Source: CAD feature listing. Evaluate the final solid. Frame: model axes, mm. Face numbers are marked on the shaded views. A direction names the side the tool comes from. Give positions to 0.01 mm unless a question says otherwise; leave off trailing zeros. Order: outer loops, then holes, each group sorted by start corner. A loop starts at its lowest first (then second) coordinate and runs counter-clockwise, first axis right, second up.
from build123d import *

# Parameters (mm, degrees)
SKETCH1_R           = 1.1
BOSS_EXTRUDE1_DEPTH = 20
SKETCH2_W           = 8.5
SKETCH2_H           = 70
SKETCH2_W_2         = 17.75
SKETCH2_H_2         = 26
BOSS_EXTRUDE2_DEPTH = 1.25
CUT_EXTRUDE1_START  = -10
CUT_EXTRUDE1_DEPTH  = 1.8


with BuildPart() as part:
    # Sketch1 → Boss-Extrude1 (new body)
    with BuildSketch(Plane(origin=(0, 0, 0), x_dir=(1, 0, 0), z_dir=(0, 1, 0))):
        with BuildLine():
            Line((-30, 0), (-30, -60))
            Line((-30, -60), (30, -60))
            Line((30, -60), (30, 0))
            ThreePointArc((30, 0), (0, 30), (-30, 0))
        make_face()
        with Locations((27.94, 0)):
            Circle(SKETCH1_R, mode=Mode.SUBTRACT)
        with Locations((-27.94, 0)):
            Circle(SKETCH1_R, mode=Mode.SUBTRACT)
        with Locations((0, 27.94)):
            Circle(SKETCH1_R, mode=Mode.SUBTRACT)
        with Locations((-27.94, -57.785)):
            Circle(SKETCH1_R, mode=Mode.SUBTRACT)
        with Locations((27.94, -57.785)):
            Circle(SKETCH1_R, mode=Mode.SUBTRACT)
        with BuildLine():
            Line((27.94, -55.785), (27.94, -2))
            ThreePointArc((27.94, -2), (25.940320377, -0.035796715), (27.868418039, 1.998718595))
            ThreePointArc((27.868418039, 1.998718595), (19.756563466, 19.756563466), (1.998718595, 27.868418039))
            ThreePointArc((1.998718595, 27.868418039), (0, 25.94), (-1.998718595, 27.868418039))
            ThreePointArc((-1.998718595, 27.868418039), (-19.756563466, 19.756563466), (-27.868418039, 1.998718595))
            ThreePointArc((-27.868418039, 1.998718595), (-25.940320377, -0.035796715), (-27.94, -2))
            Line((-27.94, -2), (-27.94, -55.785))
            ThreePointArc((-27.94, -55.785), (-26.525786438, -56.370786438), (-25.94, -57.785))
            Line((-25.94, -57.785), (25.94, -57.785))
            ThreePointArc((25.94, -57.785), (26.525786438, -56.370786438), (27.94, -55.785))
        make_face(mode=Mode.SUBTRACT)
    extrude(amount=-BOSS_EXTRUDE1_DEPTH)

    # Sketch2 → Boss-Extrude2 (add)
    with BuildSketch(Plane.XZ.offset(20)):
        with BuildLine():
            Line((30, 0), (30, 60))
            Line((30, 60), (-30, 60))
            Line((-30, 60), (-30, 0))
            ThreePointArc((-30, 0), (0, -30), (30, 0))
        make_face()
        Polygon((-7.25, 53), (-7.25, 32), (-25, 32), (-25, 55), (-7.25, 55), align=None, mode=Mode.SUBTRACT)
        with Locations((0, 15)):
            Rectangle(SKETCH2_W, SKETCH2_H, mode=Mode.SUBTRACT)
        Polygon((7.25, 53), (7.25, 32), (25, 32), (25, 55), (7.25, 55), align=None, mode=Mode.SUBTRACT)
        with Locations((16.125, 15)):
            Rectangle(SKETCH2_W_2, SKETCH2_H_2, mode=Mode.SUBTRACT)
        with BuildLine():
            Line((-7.25, -16.347418764), (-9.399268665, -23.165788322))
            ThreePointArc((-9.399268665, -23.165788322), (-20.160567843, -14.783487553), (-24.919871589, -2))
            Line((-24.919871589, -2), (-7.25, -2))
            Line((-7.25, -2), (-7.25, -16.347418764))
        make_face(mode=Mode.SUBTRACT)
        with BuildLine():
            Line((7.25, -16.347418764), (9.399268665, -23.165788322))
            ThreePointArc((9.399268665, -23.165788322), (20.160567843, -14.783487553), (24.919871589, -2))
            Line((24.919871589, -2), (7.25, -2))
            Line((7.25, -2), (7.25, -16.347418764))
        make_face(mode=Mode.SUBTRACT)
        with Locations((-16.125, 15)):
            Rectangle(SKETCH2_W_2, SKETCH2_H_2, mode=Mode.SUBTRACT)
    extrude(amount=-BOSS_EXTRUDE2_DEPTH)

    # Sketch3 → Cut-Extrude1 (cut)
    with BuildSketch(Plane(origin=(0, 0, 0), x_dir=(1, 0, 0), z_dir=(0, 1, 0)).offset(CUT_EXTRUDE1_START)):
        Polygon((2.424871131, 27.94), (1.212435565, 30.04), (-1.212435565, 30.04), (-2.424871131, 27.94), (-2.923440006, 27.076453377), (-1.212435565, 25.84), (1.212435565, 25.84), (2.664841123, 27.524359781), align=None)
        Polygon((27.94, -2.424871131), (30.04, -1.212435565), (30.04, 1.212435565), (27.94, 2.424871131), (27.29756517, 2.795781052), (25.84, 1.212435565), (25.84, -1.212435565), align=None)
        Polygon((30.28224565, -58.412602831), (29.65464282, -56.07035718), (27.312397169, -55.44275435), (25.59775435, -57.157397169), (26.22535718, -59.49964282), (28.567602831, -60.12724565), (30.909848481, -60.754848481), align=None)
        Polygon((-25.59775435, -57.157397169), (-27.312397169, -55.44275435), (-29.65464282, -56.07035718), (-30.28224565, -58.412602831), (-30.909848481, -60.754848481), (-28.567602831, -60.12724565), (-26.22535718, -59.49964282), align=None)
        Polygon((-30.04, 1.212435565), (-30.04, -1.212435565), (-27.94, -2.424871131), (-25.84, -1.212435565), (-25.84, 1.212435565), (-27.443113573, 2.711748643), (-27.94, 2.424871131), align=None)
    extrude(amount=-CUT_EXTRUDE1_DEPTH, mode=Mode.SUBTRACT)


solid = part.part
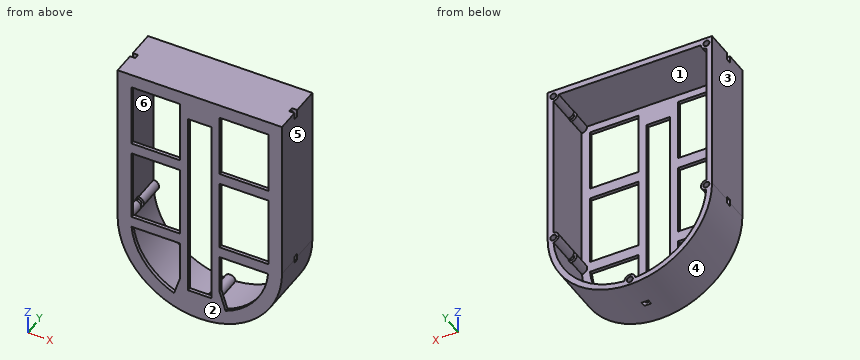
(1) Section C-C, the plane y = -5.25. Return loops of the section in (x, z) (3 decimals).
(2) Section B-B, the plane x = 0. Return loops of the section in (y, z) (3 decimals).
(3) Section D-D, the plane z = -18. Return loops of the section in (x, y), plus the area to 3 significant figures.
(4) Access query for the marked faces 5 and 6. Directions: +Z, -Z, +X, -X, +Y, -Y. A direction counts if a zero-diameter tool reaches every point of the face in a straight line with its end or side. Return the directions, or none.
(5) Line query: line 1 along X through (y, z) = (-3.25, 0); line 2 along Z through (x, y) = (0, -7.75) (3 decimals); line 3 along X through (y, z) = (-18.5, 10.5). Output: solid intervals per line, ascending.
(6) Pin query (flat end, axial travel): pin 1 Ø5.5 at (x, y) = (-2, -10.5) entering from -Z; pin 2 Ø3 at (x, z) = (-27.94, 57.785) entering from +Y; pin 3 Ø1.1 at (x, z) = (-28, 57.5) entering from +Y; pin 4 Ø2 at (x, y) = (-9.5, -6.5) entering from -Z. Return the tip coordinate at first contact, or that it passes through.
(7) Section A-A, the plane z = 13. Return loops of the section in (x, y).
(8) Draft query along X for the marked faces 1, 2, 3 and 4. Return one class per face: +X half, -X half, draft (parallel to the pull), parting line (faces both ways), or undercut.
Checks:
1. outline: (-30, 0) arc R30 ccw to (30, 0) - (30, 60) - (-30, 60) - close; hole circle Ø2.2 at (-27.94, 0); hole circle Ø2.2 at (-27.94, 57.785); hole (-27.94, 2) arc R2 cw to (-27.868, -1.999) arc R27.94 ccw to (-1.999, -27.868) arc R2 cw to (1.999, -27.868) arc R27.94 ccw to (27.868, -1.999) arc R2 cw to (27.94, 2) - (27.94, 55.785) arc R2 cw to (25.94, 57.785) - (-25.94, 57.785) arc R2 cw to (-27.94, 55.785) - close; hole circle Ø2.2 at (0, -27.94); hole circle Ø2.2 at (27.94, 0); hole circle Ø2.2 at (27.94, 57.785)
2. outline: (-20, -30) - (-11.8, -30) - (-11.8, -29.04) - (-18.75, -29.04) - (-18.75, -26.84) - (-11.8, -26.84) - (-11.8, -25.94) - (-18.75, -25.94) - (-18.75, -20) - (-20, -20) - close; (-20, 50) - (-18.75, 50) - (-18.75, 57.785) - (0, 57.785) - (0, 60) - (-20, 60) - close; (-10, -30) - (0, -30) - (0, -29.04) - (-10, -29.04) - close; (-10, -26.84) - (0, -26.84) - (0, -25.94) - (-10, -25.94) - close
3. outline: (-24, -20) - (-17.35, -20) - (-17.35, -18.75) - (-21.37, -18.75) - (-21.37, 0) - (-24, 0) - close; (-7.77, -20) - (-4.25, -20) - (-4.25, -18.75) - (-7.77, -18.75) - close; (4.25, -20) - (7.77, -20) - (7.77, -18.75) - (4.25, -18.75) - close; (17.35, -20) - (24, -20) - (24, 0) - (21.37, 0) - (21.37, -18.75) - (17.35, -18.75) - close
3. area: 124 mm2
4. face 5: +Z, -Z, +X, +Y, -Y
4. face 6: +Y
5. line 1: x = -30 to -29.04, -26.84 to -25.94, 25.94 to 26.84, 29.04 to 30
5. line 2: z = -30 to -29.04, -26.84 to -25.94, 57.785 to 60
5. line 3: x = -30 to -27.94, 27.94 to 30
6. pin 1: stops at z = -30
6. pin 2: stops at y = 0
6. pin 3: stops at y = -18.75
6. pin 4: stops at z = -28.77
7. outline: (-30, -20) - (-25, -20) - (-25, -18.75) - (-27.94, -18.75) - (-27.94, 0) - (-30, 0) - close; (-7.25, -20) - (-4.25, -20) - (-4.25, -18.75) - (-7.25, -18.75) - close; (4.25, -20) - (7.25, -20) - (7.25, -18.75) - (4.25, -18.75) - close; (25, -20) - (30, -20) - (30, 0) - (27.94, 0) - (27.94, -18.75) - (25, -18.75) - close
8. face 1: undercut
8. face 2: draft
8. face 3: -X half
8. face 4: parting line
